Read the model definition and answer for the solid it produces. Units are mm, in the model's axes. Coordinates: 2 decimals unless noted, no trailing zeros. Write each loop counter-clockwise with the first axis right and the second up, starting at its lowest first coordinate (ties: lowest second). Pieces come first, ordered by that corner, then holes.
Item 1: This flat-tipped pin is pushed along its axis until it touches: P1, Ø1.5, axis at y = -22, z = -3.5, coming from the +X side. Where does it stop, or does it pass through?
Item 2: Straight lines are drawn through the part: probe 1 along X at (y, z) = (-19.65, -12.75); probe 2 along X at (y, z) = (-20.55, -4.25); probe 3 along Z at (x, y) = (2, -21.8). For each, find the intervals that lie inside material, in ascending order.
Item 3: Section A-A (z = -8.25) is taken. Give the vertices of the cut face in (x, y), then the cut area to 3 significant figures.
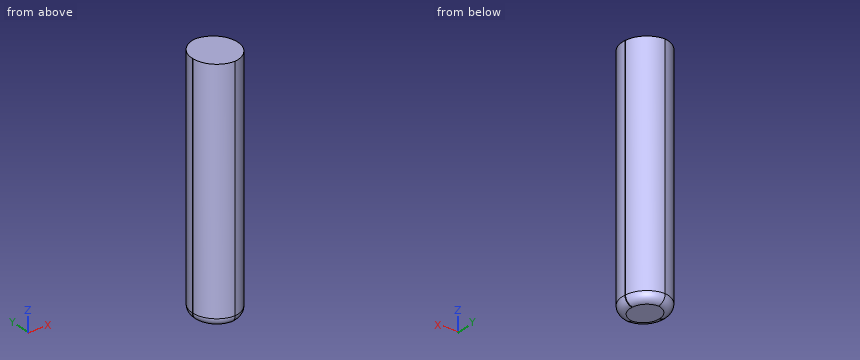
from build123d import *

# Parameters (mm, degrees)
F1_DEPTH     = 15
F2_T1_DEPTH  = 23.0140868267
F2_T3_DEPTH  = 23.0408505773
F2_T5_DEPTH  = 22.0139169115
F2_T7_DEPTH  = 22.0399446
F3_T1_DEPTH  = 0.0435766834
F3_T3_DEPTH  = 0.0435423936
F3_T6_ANGLE  = 137.6611177832
F3_T8_ANGLE  = 137.8590578992
F3_T10_ANGLE = 130.081684858
F3_T12_ANGLE = 130.2935410412


# Not quite as in the source:
# - a fillet or chamfer that OpenCascade refuses, or shapes differently, is made with other operations: its cross-section is extruded or revolved along the edge and cut away or added


with BuildPart() as f1:
    # F0 (on Top) → F1 (new body)
    with BuildSketch(Plane.XY):
        with BuildLine():
            Line((0, -19.5), (0, -22.5))
            ThreePointArc((0, -22.5), (1.5, -22.4499443206), (2.9933259094, -22.3))
            Line((2.9933259094, -22.3), (2.9438857713, -21.9224737536))
            Line((2.9438857713, -21.9224737536), (2.6037776482, -19.3253988247))
            Line((2.6037776482, -19.3253988247), (0, -19.5))
        make_face()
    extrude(amount=-F1_DEPTH)

    # F2: fillet of radius 1.5 on 4 edges, made by hand

    # F2_s2 → F2_t1 (cut)
    with BuildSketch(Plane.XY.offset(-19.0070434133)):
        with BuildLine():
            ThreePointArc((1.3981688146, -22.4565162918), (2.4625908606, -21.9132942034), (2.792258148, -20.7646410751))
            Line((2.792258148, -20.7646410751), (2.9933259094, -22.3))
            ThreePointArc((2.9933259094, -22.3), (2.1971415101, -22.3924667954), (1.3981688146, -22.4565162918))
        make_face()
    extrude(amount=F2_T1_DEPTH, mode=Mode.SUBTRACT)

    # F2_s4 → F2_t3 (cut)
    with BuildSketch(Plane.XY.offset(-19.0204252887)):
        with BuildLine():
            ThreePointArc((1.6071428571, -22.4425286418), (0.4779222842, -22.0442476477), (0, -20.9463600657))
            Line((0, -20.9463600657), (0, -22.5))
            ThreePointArc((0, -22.5), (0.8040850577, -22.4856275701), (1.6071428571, -22.4425286418))
        make_face()
    extrude(amount=F2_T3_DEPTH, mode=Mode.SUBTRACT)

    # F2_s6 → F2_t5 (cut)
    with BuildSketch(Plane.XY.offset(-18.5069584558)):
        with BuildLine():
            ThreePointArc((1.3996400846, -19.4061445189), (0.4044316833, -19.8782200297), (0, -20.9027833823))
            Line((0, -20.9027833823), (0, -19.5))
            Line((0, -19.5), (1.3996400846, -19.4061445189))
        make_face()
    extrude(amount=F2_T5_DEPTH, mode=Mode.SUBTRACT)

    # F2_s8 → F2_t7 (cut)
    with BuildSketch(Plane.XY.offset(-18.5199723)):
        with BuildLine():
            ThreePointArc((1.1989436903, -19.4196025906), (2.2504156143, -19.7563337218), (2.7866041934, -20.7214673234))
            Line((2.7866041934, -20.7214673234), (2.6037776482, -19.3253988247))
            Line((2.6037776482, -19.3253988247), (1.1989436903, -19.4196025906))
        make_face()
    extrude(amount=F2_T7_DEPTH, mode=Mode.SUBTRACT)

    # F3: fillet of radius 0.5 on 6 edges, made by hand

    # F3_s2 → F3_t1 (cut)
    with BuildSketch(Plane.XZ.offset(20.9027833823)):
        with BuildLine():
            ThreePointArc((0, -14.5), (0.1464466094, -14.8535533906), (0.5, -15))
            Line((0.5, -15), (0, -15))
            Line((0, -15), (0, -14.5))
        make_face()
    extrude(amount=F3_T1_DEPTH, mode=Mode.SUBTRACT)

    # F3_s4 → F3_t3 (cut)
    with BuildSketch(Plane(origin=(2.7205290964, -20.7740345789, 0), x_dir=(0, 0, 1), z_dir=(-0.1298494204, 0.9915337251, 0))):
        with BuildLine():
            ThreePointArc((-14.5, 0.0723415147), (-14.8535533906, -0.0741050947), (-15, -0.4276584853))
            Line((-15, -0.4276584853), (-15, 0.0723415147))
            Line((-15, 0.0723415147), (-14.5, 0.0723415147))
        make_face()
    extrude(amount=F3_T3_DEPTH, mode=Mode.SUBTRACT)

    # F3_s5 → F3_t6 (revolve, cut)
    with BuildSketch(Plane(origin=(2.7205290981, -20.7740345786, 0), x_dir=(0, 0, 1), z_dir=(-0.1298494205, 0.9915337251, 0))):
        with BuildLine():
            ThreePointArc((-14.5, 0.072341513), (-14.8535533906, -0.0741050964), (-15, -0.427658487))
            Line((-15, -0.427658487), (-15, 0.072341513))
            Line((-15, 0.072341513), (-14.5, 0.072341513))
        make_face()
    revolve(axis=Axis((1.3049575605, -20.9594152058, -15), (0, 0, -1)), revolution_arc=F3_T6_ANGLE, mode=Mode.SUBTRACT)

    # F3_s7 → F3_t8 (revolve, cut)
    with BuildSketch(Plane(origin=(-9.7457924884, -10.7704005546, 0), x_dir=(0, 0, 1), z_dir=(0.6709566447, 0.7414965819, 0))):
        with BuildLine():
            ThreePointArc((-14.5, 16.6663443409), (-14.8535533906, 16.5198977315), (-15, 16.1663443409))
            Line((-15, 16.1663443409), (-15, 16.6663443409))
            Line((-15, 16.6663443409), (-14.5, 16.6663443409))
        make_face()
    revolve(axis=Axis((1.5000000001, -20.9463600656, -15), (0, 0, -1)), revolution_arc=F3_T8_ANGLE, mode=Mode.SUBTRACT)

    # F3_s9 → F3_t10 (revolve, cut)
    with BuildSketch(Plane.XZ.offset(20.9027833823)):
        with BuildLine():
            ThreePointArc((0, -14.5), (0.1464466094, -14.8535533906), (0.5, -15))
            Line((0.5, -15), (0, -15))
            Line((0, -15), (0, -14.5))
        make_face()
    revolve(axis=Axis((1.5, -20.9027833823, -15), (0, 0, -1)), revolution_arc=F3_T10_ANGLE, mode=Mode.SUBTRACT)

    # F3_s11 → F3_t12 (revolve, cut)
    with BuildSketch(Plane(origin=(-9.8225330213, -10.8154463672, 0), x_dir=(0, 0, 1), z_dir=(-0.672309547, -0.7402701352, 0))):
        with BuildLine():
            ThreePointArc((-14.5, -13.5240244723), (-14.8535533906, -13.6704710817), (-15, -14.0240244723))
            Line((-15, -14.0240244723), (-15, -13.5240244723))
            Line((-15, -13.5240244723), (-14.5, -13.5240244723))
        make_face()
    revolve(axis=Axis((1.2993036057, -20.916241454, -15), (0, 0, -1)), revolution_arc=F3_T12_ANGLE, mode=Mode.SUBTRACT)


solid = f1.part
Established:
1. P1: stops at x = 2.78
2. probe 1: x = 0.68 to 2.1
2. probe 2: x = 0.04 to 2.75
2. probe 3: z = -14.99 to 0
3. outline: (0, -20.95) arc R1.5 ccw to (1.5, -22.45) arc R1.5 ccw to (2.79, -20.76) - (2.79, -20.72) arc R1.5 ccw to (1.3, -19.42) arc R1.5 ccw to (0, -20.9) - close
3. area: 6.60 mm2
